CAD build for the part. Positions are in the model's coordinates, mm. Face numbers are marked on the shaded views. A direction names the side the tool comes from. Coordinates: 2 decimals unless noted, no trailing zeros. Write each loop counter-clockwise with the first axis right and the second up, starting at its lowest first coordinate (ties: lowest second). Pieces come first, ordered by that corner, then holes. Notation, with made-up numbers: (13, 62.25) -> (17, 62.25) arc R11 ccw to (17, 73.25) -> close; hole circle Ø3 at (48.25, -0.75). An arc over 180 degrees is marked (long way). Answer as CSV lines item,"result".
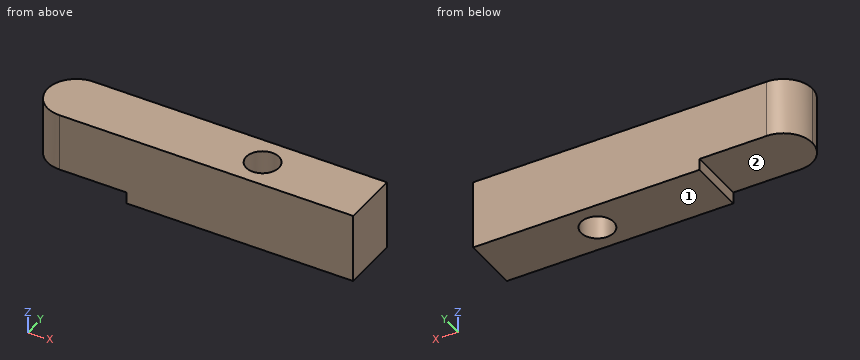
```python
from build123d import *

# Parameters (mm, degrees)
F0_W     = 84
F0_H     = 15
F1_DEPTH = 15
F3_R     = 7.49999
F4_W     = 59
F4_H     = 15
F5_DEPTH = 3
F2_R     = 4.25
F6_DEPTH = 18.001


# Not quite as in the source:
# - a fillet or chamfer is up to 0.001 mm smaller than in the source, because OpenCascade refuses the exact size


with BuildPart() as f1:
    # F0 (on Front) → F1 (new body)
    with BuildSketch(Plane.XZ):
        Rectangle(F0_W, F0_H)
    extrude(amount=-F1_DEPTH)

    # F3 (radius 7.5 in the source; OpenCascade refuses exactly that, so slightly less here)
    f3_edges = [f1.edges().sort_by_distance(p)[0] for p in [
        (-42, 15, 0),
        (-42, 0, 0),
    ]]
    fillet(f3_edges, radius=F3_R)

    # F4 (on face) → F5 (join)
    with BuildSketch(Plane(origin=(0, 0, -7.5), x_dir=(1, 0, 0), z_dir=(0, 0, -1))):
        with Locations((12.5, -7.5)):
            Rectangle(F4_W, F4_H)
    extrude(amount=F5_DEPTH)

    # F2 (on face) → F6 (cut, through all)
    with BuildSketch(Plane.XY.offset(7.5)):
        with Locations((14, 7.5)):
            Circle(F2_R)
    extrude(amount=-F6_DEPTH, mode=Mode.SUBTRACT)


solid = f1.part
```
Item 1: 3-axis set-ups, long thin cutter, end or side, ignore diameter. For the marked faces 1 and 2: which of +Z, -Z, +X, -X, +Y, -Y reach the whole face in a straight line?
Answer below:
face 1,"-Z, +X, -X, +Y, -Y"
face 2,"-Z, -X, +Y, -Y"
Item 2: Wall check: line 1 (Y direction, x = 14, z = -3.5); line 2 (Z direction, x = -33, y = 13.25); line 3 (X direction, y = 8.5, z = -5.75). Give the ranges that are in metal, low to high. Write a range as from..to.
Answer below:
line 1,"y = 0..3.25, 11.75..15"
line 2,"z = -7.5..7.5"
line 3,"x = -41.93..9.87, 18.13..42"
Item 3: Flat gauge pin, fed straight in: pin 1 (1.5 mm diameter, centred on y = 10.5, z = -9.5, fed in from -X). Where does the tip first touch, or does it go through?
Answer below:
pin 1,"stops at x = -17"
Item 4: Saw through at A-A on x = 14. Give the cut face in (y, z).
Answer below:
outline,"(0, -10.5) -> (3.25, -10.5) -> (3.25, 7.5) -> (0, 7.5) -> close; (11.75, -10.5) -> (15, -10.5) -> (15, 7.5) -> (11.75, 7.5) -> close"
Item 5: Saw through at C-C on y = 5. Give the cut face in (x, z), and give its area (3 significant figures).
Answer below:
outline,"(-41.57, -7.5) -> (-17, -7.5) -> (-17, -10.5) -> (10.56, -10.5) -> (10.56, 7.5) -> (-41.57, 7.5) -> close; (17.44, -10.5) -> (42, -10.5) -> (42, 7.5) -> (17.44, 7.5) -> close"
area,"1,310 mm2"
Item 6: Saw through at D-D on y = 13.5. Give the cut face in (x, z), and give its area (3 significant figures).
Answer below:
outline,"(-39, -7.5) -> (-17, -7.5) -> (-17, -10.5) -> (42, -10.5) -> (42, 7.5) -> (-39, 7.5) -> close"
area,"1,390 mm2"
